```python
from build123d import *

# Parameters (mm, degrees)
SKETCH1_R        = 1.984375
EXT_SHANK_DEPTH  = 13.7922
SKETCH3_R        = 2.9718
EXT_CLINCH_DEPTH = 1.9812


with BuildPart() as part:
    # Sketch1 → Ext Shank (new body)
    with BuildSketch(Plane.XY):
        Circle(SKETCH1_R)
    extrude(amount=EXT_SHANK_DEPTH)

    # Sketch2 → Rev Head (revolve)
    with BuildSketch(Plane(origin=(0, 0, 0), x_dir=(1, 0, 0), z_dir=(0, 1, 0))):
        with BuildLine():
            Line((0, 2.9718), (0, 0))
            Line((0, 0), (3.96875, 0))
            ThreePointArc((3.96875, 0), (2.479040732, 2.146511287), (0, 2.9718))
        make_face()
    revolve(axis=Axis((0, 0, 0), (0, 0, -1)))

    # Sketch3 → Ext Clinch (add)
    with BuildSketch(Plane.XY.offset(13.7922)):
        Circle(SKETCH3_R)
    extrude(amount=-EXT_CLINCH_DEPTH)


solid = part.part
```
The model under review builds one solid part; all positions refer to its coordinate system, in mm. Coordinates: 2 decimals unless noted, no trailing zeros. Write each loop counter-clockwise with the first axis right and the second up, starting at its lowest first coordinate (ties: lowest second). Pieces come first, ordered by that corner, then holes. Notation, with made-up numbers: (78, 32.5) -> (123, 32.5) arc R26 ccw to (123, 52.5) -> close; hole circle Ø9 at (88.5, -14.5). An arc over 180 degrees is marked (long way). One line per item, written item: value. Start each with the question number.
Q1. To check wall thickness, follow probe 1 along Z at (x, y) = (0, -2.25); probe 2 along Z at (x, y) = (1, 2.5); probe 3 along X at (y, z) = (-0.75, 11.75). State the ranges of each line that lie inside material, in increasing order.
Q2. Add section C-C, the plane z = 6.75. Give the boundary of the cut face in (x, y), then the cut area to 3 significant figures.
Q3. Clearance check with flat-ended pins moving along their axes: P1, Ø3, axis at x = 1.5, z = 4.5, coming from the -Y side; P2, Ø2, axis at x = -0.5, z = -1, coming from the +Y side; P3, Ø1.5, axis at x = 3, y = 3, coming from the -Z side. State where each tip first meets the part, or that it passes through.
Q4. Add section A-A, the plane x = 0. Give the boundary of the cut face in (y, z).
Q5. The part is to be moulded in two halves that separate along Z. For faces 1 (the face through (-0.43, -1.937, 5.823)), 2 (the face through (0, 0, 13.792)), 3 (the face through (2.835, 0.893, 12.815)), say which applies: +Z half, -Z half, draft (parallel to the pull), parting line (faces both ways), or undercut.
Q6. Add section D-D, the plane y = -2.5. Give the boundary of the cut face in (x, z).
Response:
1. probe 1: -2.31 to 0, 11.81 to 13.79
1. probe 2: -1.98 to 0, 11.81 to 13.79
1. probe 3: -1.84 to 1.84
2. outline: circle Ø3.97 at (0, 0)
2. area: 12.4 mm²
3. P1: y = -1.98
3. P2: y = 3.95
3. P3: z = -1.05
4. outline: (-3.97, 0) arc R4.14 ccw to (3.97, 0) -> (1.98, 0) -> (1.98, 11.81) -> (2.97, 11.81) -> (2.97, 13.79) -> (-2.97, 13.79) -> (-2.97, 11.81) -> (-1.98, 11.81) -> (-1.98, 0) -> close
5. face 1: undercut
5. face 2: +Z half
5. face 3: draft
6. outline: (-3.08, 0) arc R3.29 ccw to (3.08, 0) -> close; (-1.61, 11.81) -> (1.61, 11.81) -> (1.61, 13.79) -> (-1.61, 13.79) -> close
